from build123d import *

# Parameters (mm, degrees)
SKETCH1_W           = 75
SKETCH1_H           = 10
SKETCH1_R           = 1.518320508
BOSS_EXTRUDE1_DEPTH = 10
SKETCH5_W           = 10
SKETCH5_H           = 10
BOSS_EXTRUDE3_DEPTH = 150


with BuildPart() as part:
    # Sketch1 → Boss-Extrude1 (new body)
    with BuildSketch(Plane(origin=(0, 0, 0), x_dir=(1, 0, 0), z_dir=(0, 1, 0))):
        with Locations((37.5, 5)):
            Rectangle(SKETCH1_W, SKETCH1_H)
        with Locations(Location((5, 5, 0), (0, 0, 270))):
            Circle(SKETCH1_R, mode=Mode.SUBTRACT)
        with Locations(Location((19, 5, 0), (0, 0, 270))):
            Circle(SKETCH1_R, mode=Mode.SUBTRACT)
    extrude(amount=BOSS_EXTRUDE1_DEPTH)

    # Sketch5 → Boss-Extrude3 (add)
    with BuildSketch(Plane.XY):
        with Locations((70, 5)):
            Rectangle(SKETCH5_W, SKETCH5_H)
    extrude(amount=BOSS_EXTRUDE3_DEPTH)


solid = part.part
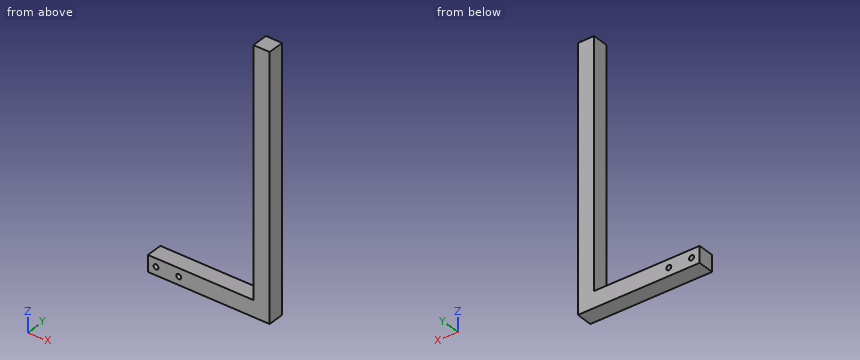
Source: CAD feature listing. Evaluate the final solid. Frame: model axes, mm. Round coordinates to 2 decimals unless told otherwise and drop trailing zeros. Write each loop counter-clockwise with the first axis right and the second up, starting at its lowest first coordinate (ties: lowest second). Pieces come first, ordered by that corner, then holes. Notation, with made-up numbers: (37, 57) - (55, 57) arc R21 ccw to (55, 85) - close; hole circle Ø9 at (-35, 65). An arc over 180 degrees is marked (long way). Use CSV: the item, a comma, the result in double quotes. Start each with the question number.
(1) First-contact query: pin 1 Ø1.5 at (x, y) = (36.5, 9) entering from +Z; pin 2 Ø3 at (y, z) = (6.5, 58.5) entering from -X; pin 3 Ø1.8 at (x, z) = (5, -5) entering from -Y. Flat tips, straight axial feed; report the tip coordinate or a pass-through.
(2) Cut plane C-C, the plane y = 5. Return loops of the section in (x, z).
(3) Cut plane A-A, the plane z = -5. Return loops of the section in (x, y), and give its area (3 significant figures).
(4) Cut plane D-D, the plane z = 41. Return loops of the section in (x, y).
(5) Material intervals for probe 1 along X at (y, z) = (5.5, -5); probe 2 along Z at (x, y) = (31, 5.75); probe 3 along X at (y, z) = (3.5, 64), sorted ascending. Write a range as [from, to].
(6) Cut plane B-B, the plane x = 5. Return loops of the section in (y, z).
Geometry says:
1,pin 1,"z = 0"
1,pin 2,"x = 65"
1,pin 3,"through"
2,outline,"(0, -10) - (75, -10) - (75, 150) - (65, 150) - (65, 0) - (0, 0) - close; hole circle Ø3.04 at (5, -5); hole circle Ø3.04 at (19, -5)"
3,outline,"(0, 0) - (3.48, 0) - (3.48, 10) - (0, 10) - close; (6.52, 0) - (17.48, 0) - (17.48, 10) - (6.52, 10) - close; (20.52, 0) - (75, 0) - (75, 10) - (20.52, 10) - close"
3,area,"689 mm²"
4,outline,"(65, 0) - (75, 0) - (75, 10) - (65, 10) - close"
5,probe 1,"[0, 3.48], [6.52, 17.48], [20.52, 75]"
5,probe 2,"[-10, 0]"
5,probe 3,"[65, 75]"
6,outline,"(0, -10) - (10, -10) - (10, -6.52) - (0, -6.52) - close; (0, -3.48) - (10, -3.48) - (10, 0) - (0, 0) - close"
